```python
from build123d import *

# Parameters (mm, degrees)
EXTRUDE_1_DEPTH     = 7
EXTRUDE_2_DEPTH     = 7
EXTRUDE_3_DEPTH     = 7
CUT_EXTRUDE_1_REACH = 122.249
SKETCH_5_R          = 1.075
CUT_EXTRUDE_2_REACH = 101.166
SKETCH_6_R          = 1.075
CUT_EXTRUDE_3_REACH = 122.249
SKETCH_7_R          = 1.075
SKETCH_8_W          = 36
SKETCH_8_H          = 16.035898384
EXTRUDE_4_DEPTH     = 7
SKETCH_9_W          = 36
SKETCH_9_H          = 20.035898384
EXTRUDE_5_DEPTH     = 5.5
SKETCH_10_R         = 1.2
CUT_EXTRUDE_4_DEPTH = 72.760416725
FILLET_1_R          = 8
SKETCH_12_W         = 8.3
SKETCH_12_H         = 24.649880383
CUT_EXTRUDE_6_DEPTH = 71.152809904
FILLET_2_R          = 1
SKETCH_13_R         = 2.5
CUT_EXTRUDE_7_DEPTH = 3
EXTRUDE_6_DEPTH     = 12.5
SKETCH_16_R         = 0.975
CUT_EXTRUDE_8_DEPTH = 20


with BuildPart() as part:
    # ｽｹｯﾁ1 → ﾎﾞｽ - 押し出し1 (new body)
    with BuildSketch(Plane(origin=(0, 0, 0), x_dir=(1, 0, 0), z_dir=(0, 1, 0))):
        Polygon((-18, -33.197640478), (18, -33.197640478), (18, -35.197640478), (37.954700538, -35.197640478), (49.459401077, -15.27091462), (39.482050808, 2.010362971), (37.75, 1.010362971), (19.75, 32.187277507), (21.482050808, 33.187277507), (11.504700538, 50.468555098), (-11.504700538, 50.468555098), (-21.482050808, 33.187277507), (-19.75, 32.187277507), (-37.75, 1.010362971), (-39.482050808, 2.010362971), (-49.459401077, -15.27091462), (-37.954700538, -35.197640478), (-18, -35.197640478), align=None)
        Polygon((-10.35, 48.468555098), (10.35, 48.468555098), (18.75, 33.919328315), (17.017949192, 32.919328315), (37.017949192, -1.721687836), (38.75, -0.721687836), (47.15, -15.27091462), (36.8, -33.197640478), (20, -33.197640478), (20, -31.197640478), (-20, -31.197640478), (-20, -33.197640478), (-36.8, -33.197640478), (-47.15, -15.27091462), (-38.75, -0.721687836), (-37.017949192, -1.721687836), (-17.017949192, 32.919328315), (-18.75, 33.919328315), align=None, mode=Mode.SUBTRACT)
    extrude(amount=EXTRUDE_1_DEPTH)

    # ｽｹｯﾁ3 → ﾎﾞｽ - 押し出し2 (add)
    with BuildSketch(Plane.XZ):
        Polygon((-20, 13.697640478), (-20, 31.197640478), (-18, 31.197640478), (-18, 15.161742094), (18, 15.161742094), (18, 31.197640478), (20, 31.197640478), (20, 13.697640478), (21.862504626, 10.471687836), (37.017949192, 1.721687836), (36.017949192, -0.010362971), (22.130453819, 8.007586221), (4.130453819, -23.169328315), (18.017949192, -31.187277507), (17.017949192, -32.919328315), (1.862504626, -24.169328315), (-1.862504626, -24.169328315), (-17.017949192, -32.919328315), (-18.017949192, -31.187277507), (-4.130453819, -23.169328315), (-22.130453819, 8.007586221), (-36.017949192, -0.010362971), (-37.017949192, 1.721687836), (-21.862504626, 10.471687836), align=None)
        Polygon((-20.398403011, 9.007586221), (-18, 13.161742094), (18, 13.161742094), (20.398403011, 9.007586221), (2.398403011, -22.169328315), (-2.398403011, -22.169328315), align=None, mode=Mode.SUBTRACT)
    extrude(amount=-EXTRUDE_2_DEPTH)

    # ｽｹｯﾁ4 → ﾎﾞｽ - 押し出し3 (add)
    with BuildSketch(Plane.XZ):
        Polygon((31.026497308, 33.197640478), (33.819872981, 28.359371888), (38.15, 30.859371888), (39.15, 29.127321081), (34.819872981, 26.627321081), (40.469872981, 16.841234018), (44.8, 19.341234018), (45.8, 17.60918321), (41.469872981, 15.10918321), (44.263248654, 10.27091462), (43.108548116, 8.27091462), (37.844074487, 17.389250421), (23.862504626, 9.316987298), (21.862504626, 10.471687836), (36.844074487, 19.121301228), (34.98156986, 22.34725387), (20, 13.697640478), (20, 16.007041555), (33.98156986, 24.079304678), (28.717096231, 33.197640478), align=None)
        Polygon((-31.026497308, 33.197640478), (-28.717096231, 33.197640478), (-33.98156986, 24.079304678), (-20, 16.007041555), (-20, 13.697640478), (-34.98156986, 22.34725387), (-36.844074487, 19.121301228), (-21.862504626, 10.471687836), (-23.862504626, 9.316987298), (-37.844074487, 17.389250421), (-43.108548116, 8.27091462), (-44.263248654, 10.27091462), (-41.469872981, 15.10918321), (-45.8, 17.60918321), (-44.8, 19.341234018), (-40.469872981, 16.841234018), (-34.819872981, 26.627321081), (-39.15, 29.127321081), (-38.15, 30.859371888), (-33.819872981, 28.359371888), align=None)
        Polygon((-14.391451884, -41.468555098), (-3.862504626, -41.468555098), (-3.862504626, -25.324028853), (-1.862504626, -24.169328315), (-1.862504626, -41.468555098), (1.862504626, -41.468555098), (1.862504626, -24.169328315), (3.862504626, -25.324028853), (3.862504626, -41.468555098), (14.391451884, -41.468555098), (13.236751346, -43.468555098), (7.65, -43.468555098), (7.65, -48.468555098), (5.65, -48.468555098), (5.65, -43.468555098), (-5.65, -43.468555098), (-5.65, -48.468555098), (-7.65, -48.468555098), (-7.65, -43.468555098), (-13.236751346, -43.468555098), align=None)
    extrude(amount=-EXTRUDE_3_DEPTH)

    # ｶｯﾄ - 押し出し1: up to this face of the body (flat: up to its plane)
    cut_extrude_1_end = Plane(part.part.faces().sort_by_distance((19.199201506, 3.5, 11.084664157))[0])
    # ｽｹｯﾁ5 → ｶｯﾄ - 押し出し1 (cut, up to the picked face)
    with BuildSketch(Plane(origin=(43.707050808, 0, 25.234277549), x_dir=(0.5, 0, -0.8660254037844386), z_dir=(0.8660254037844387, 0, 0.5000000000000001)), mode=Mode.PRIVATE) as cut_extrude_1_sk1:
        with Locations((0, 3.5)):
            Circle(SKETCH_5_R)
    cut_extrude_1_tool1 = split(extrude(cut_extrude_1_sk1.sketch, amount=-CUT_EXTRUDE_1_REACH, mode=Mode.PRIVATE), bisect_by=cut_extrude_1_end, keep=Keep.BOTH, mode=Mode.PRIVATE)
    add(cut_extrude_1_tool1.solids().sort_by(Axis((43.707051, 3.5, 25.234278), (-0.8660254037844387, 0, -0.5000000000000001)))[0], mode=Mode.SUBTRACT)

    # ｶｯﾄ - 押し出し2: up to this face of the body (flat: up to its plane)
    cut_extrude_2_end = Plane(part.part.faces().sort_by_distance((0, 3.5, -22.169328315))[0])
    # ｽｹｯﾁ6 → ｶｯﾄ - 押し出し2 (cut, up to the picked face)
    with BuildSketch(Plane(origin=(0, 0, -50.468555098), x_dir=(-1, 0, 0), z_dir=(0, 0, -1)), mode=Mode.PRIVATE) as cut_extrude_2_sk1:
        with Locations((0, 3.5)):
            Circle(SKETCH_6_R)
    cut_extrude_2_tool1 = split(extrude(cut_extrude_2_sk1.sketch, amount=-CUT_EXTRUDE_2_REACH, mode=Mode.PRIVATE), bisect_by=cut_extrude_2_end, keep=Keep.BOTH, mode=Mode.PRIVATE)
    add(cut_extrude_2_tool1.solids().sort_by(Axis((0, 3.5, -50.468555), (0, 0, 1)))[0], mode=Mode.SUBTRACT)

    # ｶｯﾄ - 押し出し3: up to this face of the body (flat: up to its plane)
    cut_extrude_3_end = Plane(part.part.faces().sort_by_distance((-19.199201506, 3.5, 11.084664157))[0])
    # ｽｹｯﾁ7 → ｶｯﾄ - 押し出し3 (cut, up to the picked face)
    with BuildSketch(Plane(origin=(-43.707050808, 0, 25.234277549), x_dir=(0.5000000000000001, 0, 0.8660254037844386), z_dir=(-0.8660254037844386, 0, 0.5000000000000001)), mode=Mode.PRIVATE) as cut_extrude_3_sk1:
        with Locations((0, 3.5)):
            Circle(SKETCH_7_R)
    cut_extrude_3_tool1 = split(extrude(cut_extrude_3_sk1.sketch, amount=-CUT_EXTRUDE_3_REACH, mode=Mode.PRIVATE), bisect_by=cut_extrude_3_end, keep=Keep.BOTH, mode=Mode.PRIVATE)
    add(cut_extrude_3_tool1.solids().sort_by(Axis((-43.707051, 3.5, 25.234278), (0.8660254037844386, 0, -0.5000000000000001)))[0], mode=Mode.SUBTRACT)

    # ｽｹｯﾁ8 → ﾎﾞｽ - 押し出し4 (add)
    with BuildSketch(Plane(origin=(0, 7, 0), x_dir=(1, 0, 0), z_dir=(0, 1, 0))):
        with Locations((0, -23.179691286)):
            Rectangle(SKETCH_8_W, SKETCH_8_H)
    extrude(amount=-EXTRUDE_4_DEPTH)

    # ｽｹｯﾁ9 → ﾎﾞｽ - 押し出し5 (add)
    with BuildSketch(Plane(origin=(0, 7, 0), x_dir=(1, 0, 0), z_dir=(0, 1, 0))):
        with Locations((0, -23.179691286)):
            Rectangle(SKETCH_9_W, SKETCH_9_H)
    extrude(amount=EXTRUDE_5_DEPTH)

    # ｽｹｯﾁ10 → ｶｯﾄ - 押し出し4 (cut, through all)
    with BuildSketch(Plane(origin=(0, 12.5, 0), x_dir=(1, 0, 0), z_dir=(0, 1, 0))):
        with Locations(Location((-11.5, -28.897640478, 0), (0, 0, 270))):
            Circle(SKETCH_10_R)
        with Locations(Location((11.5, -28.897640478, 0), (0, 0, 270))):
            Circle(SKETCH_10_R)
    extrude(amount=-CUT_EXTRUDE_4_DEPTH, mode=Mode.SUBTRACT)

    # ﾌｨﾚｯﾄ1
    fillet_1_edges = [part.edges().sort_by_distance(p)[0] for p in [
        (-49.459401077, 3.5, 15.27091462),
        (49.459401077, 3.5, 15.27091462),
    ]]
    fillet(fillet_1_edges, radius=FILLET_1_R)

    # ｽｹｯﾁ12 → ｶｯﾄ - 押し出し6 (cut, through all)
    with BuildSketch(Plane(origin=(0, 7, 0), x_dir=(1, 0, 0), z_dir=(0, 1, 0))):
        with Locations((-50, -9.197640479)):
            Rectangle(SKETCH_12_W, SKETCH_12_H)
        with Locations((50, -9.197640479)):
            Rectangle(SKETCH_12_W, SKETCH_12_H)
    extrude(amount=-CUT_EXTRUDE_6_DEPTH, mode=Mode.SUBTRACT)

    # ﾌｨﾚｯﾄ2
    fillet_2_edges = [part.edges().sort_by_distance(p)[0] for p in [
        (42.666025404, 7, 3.5044428),
        (45.85, 3.5, 9.01924857),
        (45.85, 7, 11.01924857),
        (45.85, 7, 19.52258067),
        (45.85, 3.5, 21.52258067),
        (41.902350269, 7, 28.360110574),
        (-41.902350269, 7, 28.360110574),
        (-45.85, 7, 19.52258067),
        (-45.85, 3.5, 21.52258067),
        (-45.85, 3.5, 9.01924857),
        (-42.666025404, 7, 3.5044428),
        (-45.85, 7, 11.01924857),
    ]]
    fillet(fillet_2_edges, radius=FILLET_2_R)

    # ｽｹｯﾁ13 → ｶｯﾄ - 押し出し7 (cut)
    with BuildSketch(Plane.XZ):
        with Locations(Location((11.5, 28.897640478, 0), (0, 0, 270))):
            Circle(SKETCH_13_R)
        with Locations(Location((-11.5, 28.897640478, 0), (0, 0, 270))):
            Circle(SKETCH_13_R)
    extrude(amount=-CUT_EXTRUDE_7_DEPTH, mode=Mode.SUBTRACT)

    # ｽｹｯﾁ15 → ﾎﾞｽ - 押し出し6 (add)
    with BuildSketch(Plane.XZ):
        Polygon((2.398403011, -22.169328315), (4.707804088, -18.169328315), (-4.707804088, -18.169328315), (-2.398403011, -22.169328315), align=None)
    extrude(amount=-EXTRUDE_6_DEPTH)

    # ｽｹｯﾁ16 → ｶｯﾄ - 押し出し8 (cut)
    with BuildSketch(Plane.XY.offset(35.197640478)):
        with Locations(Location((-25, 3.5, 0), (0, 0, 180))):
            Circle(SKETCH_16_R)
        with Locations((25, 3.5)):
            Circle(SKETCH_16_R)
    extrude(amount=-CUT_EXTRUDE_8_DEPTH, mode=Mode.SUBTRACT)


solid = part.part
```
Can you work these out from the model? Positions are in its coordinate system, mm. A direction names the side the tool comes from. Round coordinates to 2 decimals unless told otherwise and drop trailing zeros. Loops run counter-clockwise (first coordinate to the right, second up) from the corner with the lowest first, then second, coordinate; pieces in that order, holes last. Notation, with made-up numbers: (85.25, -1.75) -> (114.25, -1.75) arc R21 cw to (114.25, 5.25) -> close; hole circle Ø5 at (9.5, 19.5). An arc over 180 degrees is marked (long way). Answer in a Markdown table with one row per item.
Item 1: We'd pull the mould along Y, two halves only. Please class faces 1 (the flat face through (42.85, 3.45, 12.72)), 2 (the cylindrical face through (25.9, 3.13, 34.21)): released by +Y, released by -Y, zero draft, split by the parting line, or undercut.
Answer block:
| item | result |
|---|---|
| face 1 | zero draft |
| face 2 | undercut |
Item 2: On a 3-axis mill with a long thin cutter (end or side, diameter ignored), from which of +Z, -Z, +X, -X, +Y, -Y can I reach the whole of each face in a straight line? I mean faces 3 (the flat face through (18, 3, 34)), 4 (the flat face through (1.3, 3.5, -24.169)), 5 (the cylindrical face through (20.007, 4.566, 11.713)), 6 (the flat face through (45.85, 3, 19)), 7 (the cylindrical face through (0.14, 4.566, -49.483)). Say none if no direction works.
Answer block:
| item | result |
|---|---|
| face 3 | +Z, +Y, -Y |
| face 4 | +Y, -Y |
| face 5 | none |
| face 6 | +Z, -Z, +X, +Y, -Y |
| face 7 | -Z |
Item 3: Suppose I cut it at B-B, the plane z = -9. List the corners of the cut face in (x, y) for me.
Answer block:
| item | result |
|---|---|
| outline | (-33.14, 0) -> (-30.83, 0) -> (-30.83, 7) -> (-33.14, 7) -> close; (-12.31, 0) -> (-10, 0) -> (-10, 7) -> (-12.31, 7) -> close; (10, 0) -> (12.31, 0) -> (12.31, 7) -> (10, 7) -> close; (30.83, 0) -> (33.14, 0) -> (33.14, 7) -> (30.83, 7) -> close |
Item 4: If I drill on probe 1 along Y at (x, z) = (25, 18.3) (3 decimals); probe 2 along X at (y, z) = (6.75, -13); probe 3 along Z at (x, y) = (33, 4), over which ranges is the centre line in solid material (lowest first)?
Answer block:
| item | result |
|---|---|
| probe 1 | 0 to 2.525, 4.475 to 7 |
| probe 2 | -30.83 to -28.52, -10 to -7.69, 7.69 to 10, 28.52 to 30.83 |
| probe 3 | -9.24 to -5.24, 1.73 to 4.04, 14.59 to 16.9, 21.2 to 23.51, 25.78 to 29.78, 33.2 to 35.2 |
Item 5: Suppose I cut it at A-A, the plane x = 0. Give the number of separate pieces and of enclosed holes in the cut face, plus the area to 3 significant figures.
Answer block:
| item | result |
|---|---|
| separate pieces | 6 |
| enclosed holes | 0 |
| area | 330 mm² |
Item 6: Will these pins go through, and if not, where does the flat tip stop? P1, Ø3, axis at x = 11.5, z = 28.9, coming from the +Y side; P2, Ø6, axis at x = 14.5, z = -23, coming from the -Y side (1 decimal); P3, Ø6, axis at x = 13, y = 10.5, coming from the -Z side; P4, Ø1.7, axis at x = 34.5, y = 4, coming from the -Z side.
Answer block:
| item | result |
|---|---|
| P1 | y = 12.5 |
| P2 | through |
| P3 | z = 13.16 |
| P4 | z = -8.11 |
